Part model, mm, in its own coordinate system. Face numbers are marked on the shaded views. A direction names the side the tool comes from. Give positions to 0.01 mm unless a question says otherwise; leave off trailing zeros. Loops run counter-clockwise (first coordinate to the right, second up) from the corner with the lowest first, then second, coordinate; pieces in that order, holes last. Notation, with made-up numbers: M 23,77.25 L 80,77.25 A23 cw 80,93.25 Z; hole C 37,77 d7. An arc over 180 degrees is marked long. Put each result on its own line as item: value. Start each with the question number.
```python
from build123d import *

# Parameters (mm, degrees)
SKETCH1_R           = 19.9
BOSS_EXTRUDE1_DEPTH = 6
SKETCH2_R           = 22
BOSS_EXTRUDE2_DEPTH = 1
SKETCH3_R           = 2
SKETCH3_R_2         = 1.75
CUT_EXTRUDE1_DEPTH  = 32.890437438
SKETCH5_R           = 2.75
SKETCH5_R_2         = 1.75
CUT_EXTRUDE2_DEPTH  = 3
CHAMFER1_SIZE       = 1


with BuildPart() as part:
    # Sketch1 → Boss-Extrude1 (new body)
    with BuildSketch(Plane(origin=(0, 0, 0), x_dir=(1, 0, 0), z_dir=(0, 1, 0))):
        with Locations(Location((0, 0, 0), (0, 0, 270))):
            Circle(SKETCH1_R)
    extrude(amount=BOSS_EXTRUDE1_DEPTH)

    # Sketch2 → Boss-Extrude2 (add)
    with BuildSketch(Plane(origin=(0, 6, 0), x_dir=(1, 0, 0), z_dir=(0, 1, 0))):
        with Locations(Location((0, 0, 0), (0, 0, 270))):
            Circle(SKETCH2_R)
    extrude(amount=BOSS_EXTRUDE2_DEPTH)

    # Sketch3 → Cut-Extrude1 (cut, through all)
    with BuildSketch(Plane(origin=(0, 7, 0), x_dir=(1, 0, 0), z_dir=(0, 1, 0))):
        with Locations(Location((0, 17, 0), (0, 0, 270))):
            Circle(SKETCH3_R)
        with Locations(Location((17, 0, 0), (0, 0, 270))):
            Circle(SKETCH3_R)
        with Locations(Location((0, -17, 0), (0, 0, 270))):
            Circle(SKETCH3_R)
        with Locations(Location((-17, 0, 0), (0, 0, 270))):
            Circle(SKETCH3_R)
        with Locations(Location((-12.02081528, 12.02081528, 0), (0, 0, 270))):
            Circle(SKETCH3_R_2)
        with Locations(Location((12.02081528, 12.02081528, 0), (0, 0, 270))):
            Circle(SKETCH3_R_2)
        with Locations(Location((12.02081528, -12.02081528, 0), (0, 0, 270))):
            Circle(SKETCH3_R_2)
        with Locations(Location((-12.02081528, -12.02081528, 0), (0, 0, 270))):
            Circle(SKETCH3_R_2)
    extrude(amount=-CUT_EXTRUDE1_DEPTH, mode=Mode.SUBTRACT)

    # Sketch5 → Cut-Extrude2 (cut)
    # profile 1 of 4: a face of its own
    with BuildSketch(Plane(origin=(0, 7, 0), x_dir=(1, 0, 0), z_dir=(0, 1, 0))):
        with Locations(Location((-12.02081528, 12.02081528, 0), (0, 0, 270))):
            Circle(SKETCH5_R)
        with Locations(Location((-12.02081528, 12.02081528, 0), (0, 0, 270))):
            Circle(SKETCH5_R_2, mode=Mode.SUBTRACT)
    # profile 2 of 4: a face of its own
    with BuildSketch(Plane(origin=(0, 7, 0), x_dir=(1, 0, 0), z_dir=(0, 1, 0))):
        with Locations(Location((12.02081528, 12.02081528, 0), (0, 0, 270))):
            Circle(SKETCH5_R)
        with Locations(Location((12.02081528, 12.02081528, 0), (0, 0, 270))):
            Circle(SKETCH5_R_2, mode=Mode.SUBTRACT)
    # profile 3 of 4: a face of its own
    with BuildSketch(Plane(origin=(0, 7, 0), x_dir=(1, 0, 0), z_dir=(0, 1, 0))):
        with Locations(Location((12.02081528, -12.02081528, 0), (0, 0, 270))):
            Circle(SKETCH5_R)
        with Locations(Location((12.02081528, -12.02081528, 0), (0, 0, 270))):
            Circle(SKETCH5_R_2, mode=Mode.SUBTRACT)
    # profile 4 of 4: a face of its own
    with BuildSketch(Plane(origin=(0, 7, 0), x_dir=(1, 0, 0), z_dir=(0, 1, 0))):
        with Locations(Location((-12.02081528, -12.02081528, 0), (0, 0, 270))):
            Circle(SKETCH5_R)
        with Locations(Location((-12.02081528, -12.02081528, 0), (0, 0, 270))):
            Circle(SKETCH5_R_2, mode=Mode.SUBTRACT)
    extrude(amount=-CUT_EXTRUDE2_DEPTH, mode=Mode.SUBTRACT)

    # Chamfer1
    # the kernel refuses this chamfer: 1 mm, written as the material it takes off along each edge
    with BuildSketch(Plane(origin=(0, 0, 0), x_dir=(0, 0, 1), z_dir=(-1, 0, 0))) as chamfer1_piece_1:
        Polygon((19.9, CHAMFER1_SIZE), (19.9 - CHAMFER1_SIZE, 0), (19.9, 0), align=None)
    revolve(axis=Axis((0, 0, 0), (0, 1, 0)), mode=Mode.SUBTRACT)


solid = part.part
```
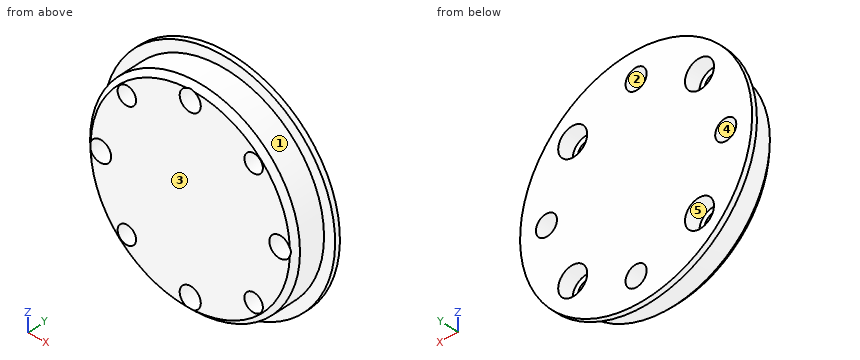
1) Band-saw the part on A-A on z = 0. Give the cut face in (x, y).
2) Mould opens along X. For the marked faces 1, 2 and 3 say: +X half, -X half, draft (parallel to the pull), parting line (faces both ways), or undercut.
3) Band-saw the part on C-C on y = 2.25. State how many separate pieces and enclosed holes the cut face has, then the cut area to 3 significant figures.
4) Wall check: L1, parallel to X at y = 1.5, z = -10.5 (3 decimals); L2, parallel to Z at x = -13.5, y = 5.25; L3, parallel to Z at x = 1, y = 4.5. Give the ranges that are in metal, low to high.
5) Band-saw the part on B-B on x = 0. Give the cut face in (y, z).
6) Pin check, flat tips, straight feed: pin 1 Ø3 at (x, z) = (13, 12) entering from +Y; pin 2 Ø4 at (x, y) = (-10, 0.5) entering from -Z; pin 3 Ø1.5 at (y, z) = (3, 1.5) entering from +X. Stop position of each tip, or through.
7) Which spindle directions (+Z, -Z, +X, -X, +Y, -Y) get a long thin tool onto all of the face, cutting with end or side? Do the marked faces 4 and 5. Say none if no direction does.
Evaluation:
1. outline: M -22,6 L -19.9,6 L -19.9,1 L -19,0.1 L -19,7 L -22,7 Z; M -15,0 L 15,0 L 15,7 L -15,7 Z; M 19,0.1 L 19.9,1 L 19.9,6 L 22,6 L 22,7 L 19,7 Z
2. face 1: parting line
2. face 2: undercut
2. face 3: draft
3. separate pieces: 1
3. enclosed holes: 8
3. area: 1,160 mm2
4. L1: -16.904 to -12.887, -11.155 to 11.155, 12.887 to 16.904
4. L2: -14.62 to -14.34, -9.7 to 9.7, 14.34 to 14.62
4. L3: -19.87 to -18.73, -15.27 to 15.27, 18.73 to 19.87
5. outline: M 0,-15 L 7,-15 L 7,15 L 0,15 Z; M 0.1,-19 L 1,-19.9 L 6,-19.9 L 6,-22 L 7,-22 L 7,-19 Z; M 0.1,19 L 7,19 L 7,22 L 6,22 L 6,19.9 L 1,19.9 Z
6. pin 1: y = 4
6. pin 2: z = -18.19
6. pin 3: x = 19.89
7. face 4: +Y, -Y
7. face 5: +Y
